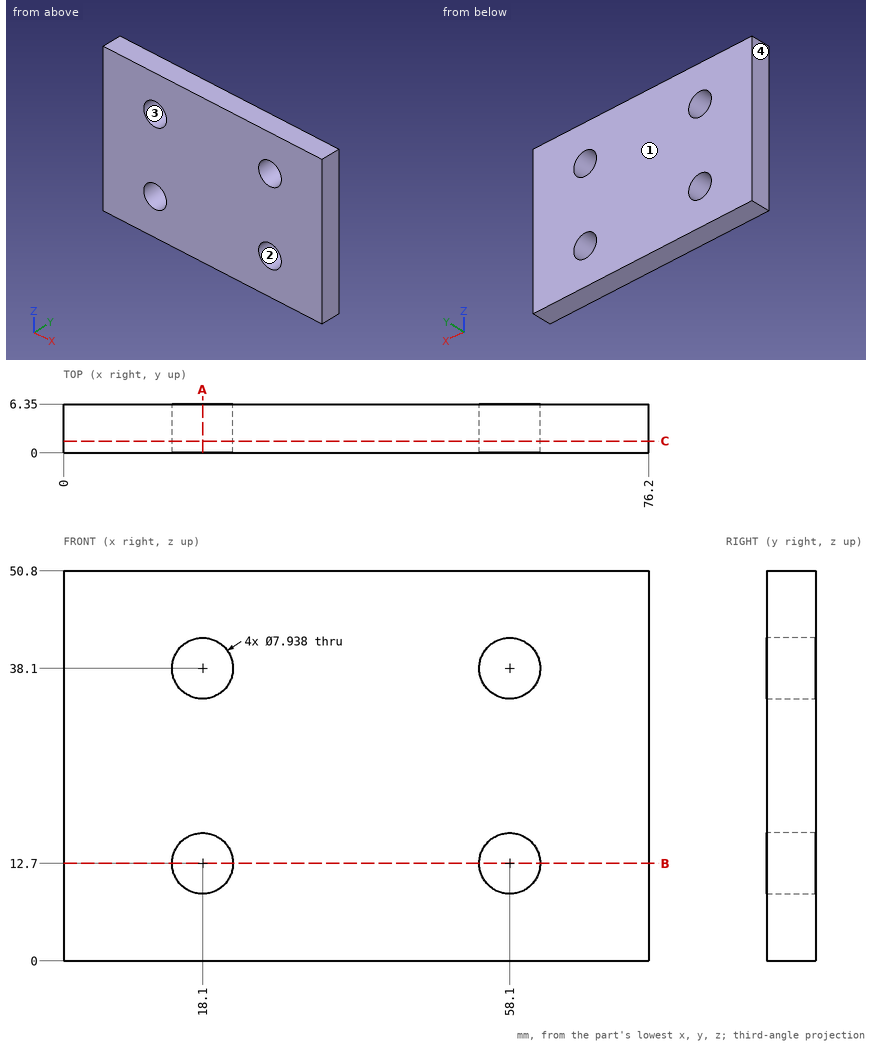
Verification items for this drawing (mm, ordinates from the low corner). Round coordinates to 2 decimals unless told otherwise and drop trailing zeros. Loops run counter-clockwise (first coordinate to the right, second up) from the corner with the lowest first, then second, coordinate; pieces in that order, holes last. Notation, with made-up numbers: M -23.75,-31.75 L 32.25,-31.75 A13 cw 32.25,-25.75 Z; hole C -22.75,-38.5 d10. An arc over 180 degrees is marked long. Answer as a JSON object with one key per item and string values.
1. Section check A-A (x = 18.1). Record the boundary of the cut face in (y, z).
Reply:
{"outline": "M 0,0 L 6.35,0 L 6.35,8.73 L 0,8.73 Z; M 0,16.67 L 6.35,16.67 L 6.35,34.13 L 0,34.13 Z; M 0,42.07 L 6.35,42.07 L 6.35,50.8 L 0,50.8 Z"}
2. Section check C-C (y = 1.5). Record the boundary of the cut face in (x, z).
Reply:
{"outline": "M 0,0 L 76.2,0 L 76.2,50.8 L 0,50.8 Z; hole C 18.1,12.7 d7.94; hole C 18.1,38.1 d7.94; hole C 58.1,12.7 d7.94; hole C 58.1,38.1 d7.94"}
3. Section check B-B (z = 12.7). Record the boundary of the cut face in (x, y), plus the area to 3 significant figures.
Reply:
{"outline": "M 0,0 L 14.13,0 L 14.13,6.35 L 0,6.35 Z; M 22.07,0 L 54.13,0 L 54.13,6.35 L 22.07,6.35 Z; M 62.07,0 L 76.2,0 L 76.2,6.35 L 62.07,6.35 Z", "area": "383 mm²"}
4. Scan lines: line 1 (X direction, y = 4, z = 38.1); line 2 (X direction, y = 4.5, z = 37); line 3 (Z direction, x = 58.5, y = 1). Record each from-to range of solid material in increasing order.
Reply:
{"line 1": "x = 0 to 14.13, 22.07 to 54.13, 62.07 to 76.2", "line 2": "x = 0 to 14.29, 21.91 to 54.29, 61.91 to 76.2", "line 3": "z = 0 to 8.75, 16.65 to 34.15, 42.05 to 50.8"}
5. Mould release check, pull along X, two halves, no side actions. Record for the marked faces 1, 2, 3 and 4: pulls with the +X half, pulls with the -X half, needs draft (parallel to the pull), parting line crosses it, or undercut.
Reply:
{"face 1": "needs draft", "face 2": "undercut", "face 3": "undercut", "face 4": "pulls with the -X half"}
6. Gauge pin test, flat ends, axial feed: P1, Ø8, axis at x = 12, z = 45, coming from the -Y side; P2, Ø5, axis at x = 58.1, z = 12.7, coming from the +Y side. Record the tip position at first contact, or that the pin passes through.
Reply:
{"P1": "stops at y = 0", "P2": "passes through"}
